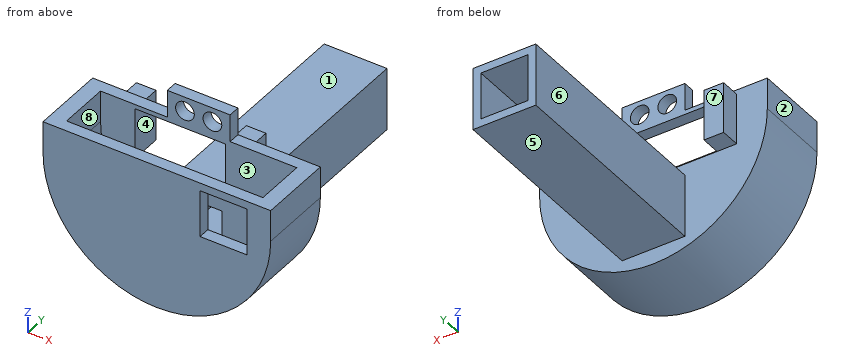
from build123d import *

# Parameters (mm, degrees)
BOSS_EXTRUDE1_DEPTH = 16
SKETCH2_5_W         = 12
SKETCH2_5_H         = 12
BOSS_EXTRUDE2_DEPTH = 3
SKETCH3_R           = 2.38125
SKETCH3_W           = 23
SKETCH3_H           = 13
SKETCH3_W_2         = 12
SKETCH3_H_2         = 12
BOSS_EXTRUDE3_DEPTH = 3
SKETCH3_4_W         = 16
SKETCH3_4_H         = 16
SKETCH3_4_W_2       = 12
SKETCH3_4_H_2       = 12
BOSS_EXTRUDE4_DEPTH = 60
SKETCH3_5_W         = 5
SKETCH3_5_H         = 13
BOSS_EXTRUDE5_DEPTH = 8


with BuildPart() as part:
    # Sketch2 → Boss-Extrude1 (new body)
    with BuildSketch(Plane(origin=(0, 0, 0), x_dir=(1, 0, 0), z_dir=(0, 1, 0))):
        with BuildLine():
            Line((25, 8), (25, 0))
            Line((25, 0), (29, 0))
            Line((29, 0), (29, 8))
            ThreePointArc((29, 8), (0, 37), (-29, 8))
            Line((-29, 8), (-29, 0))
            Line((-29, 0), (-25, 0))
            Line((-25, 0), (-25, 8))
            ThreePointArc((-25, 8), (0, 33), (25, 8))
        make_face()
    extrude(amount=BOSS_EXTRUDE1_DEPTH)

    # Sketch2_5 → Boss-Extrude2 (add)
    # profile 1 of 2: a face of its own
    with BuildSketch(Plane(origin=(0, 0, 0), x_dir=(1, 0, 0), z_dir=(0, 1, 0))):
        with BuildLine():
            ThreePointArc((-25, 8), (0, 33), (25, 8))
            Line((25, 8), (25, 0))
            Line((25, 0), (-25, 0))
            Line((-25, 0), (-25, 8))
        make_face()
        with Locations((0, 25)):
            Rectangle(SKETCH2_5_W, SKETCH2_5_H, mode=Mode.SUBTRACT)
        with Locations((17, 8)):
            Rectangle(SKETCH2_5_W, SKETCH2_5_H, mode=Mode.SUBTRACT)
    # profile 2 of 2: a face of its own
    with BuildSketch(Plane(origin=(0, 0, 0), x_dir=(1, 0, 0), z_dir=(0, 1, 0))):
        with Locations((0, 25)):
            Rectangle(SKETCH2_5_W, SKETCH2_5_H)
    extrude(amount=BOSS_EXTRUDE2_DEPTH)

    # Sketch3 → Boss-Extrude3 (add)
    with BuildSketch(Plane(origin=(0, 16, 0), x_dir=(1, 0, 0), z_dir=(0, 1, 0))):
        with BuildLine():
            Line((-29, 8), (-29, 0))
            Line((-29, 0), (-8, 0))
            Line((-8, 0), (-8, -7))
            Line((-8, -7), (8, -7))
            Line((8, -7), (8, 0))
            Line((8, 0), (29, 0))
            Line((29, 0), (29, 8))
            ThreePointArc((29, 8), (0, 37), (-29, 8))
        make_face()
        with Locations(Location((-3.5, -3.4, 0), (0, 0, 270))):
            Circle(SKETCH3_R, mode=Mode.SUBTRACT)
        with Locations(Location((3.5, -3.4, 0), (0, 0, 90))):
            Circle(SKETCH3_R, mode=Mode.SUBTRACT)
        with Locations((-4.7, 7.6)):
            Rectangle(SKETCH3_W, SKETCH3_H, mode=Mode.SUBTRACT)
        with Locations((0, 25)):
            Rectangle(SKETCH3_W_2, SKETCH3_H_2, mode=Mode.SUBTRACT)
    extrude(amount=BOSS_EXTRUDE3_DEPTH)

    # Sketch3_4 → Boss-Extrude4 (add)
    with BuildSketch(Plane(origin=(0, 16, 0), x_dir=(1, 0, 0), z_dir=(0, 1, 0))):
        with Locations((0, 25)):
            Rectangle(SKETCH3_4_W, SKETCH3_4_H)
        with Locations((0, 25)):
            Rectangle(SKETCH3_4_W_2, SKETCH3_4_H_2, mode=Mode.SUBTRACT)
    extrude(amount=BOSS_EXTRUDE4_DEPTH)

    # Sketch3_5 → Boss-Extrude5 (add)
    with BuildSketch(Plane(origin=(0, 16, 0), x_dir=(1, 0, 0), z_dir=(0, 1, 0))):
        with Locations((-18.7, 7.6)):
            Rectangle(SKETCH3_5_W, SKETCH3_5_H)
        with Locations((9.3, 7.6)):
            Rectangle(SKETCH3_5_W, SKETCH3_5_H)
    extrude(amount=BOSS_EXTRUDE5_DEPTH)


solid = part.part
For this review, take the finished solid that the model builds, in its own axes (mm). Face numbers are marked on the shaded views. A direction names the side the tool comes from. Give positions to 0.01 mm unless a question says otherwise; leave off trailing zeros. Order: outer loops, then holes, each group sorted by start corner. A loop starts at its lowest first (then second) coordinate and runs counter-clockwise, first axis right, second up. Notation, with made-up numbers: (-22, -3.5) -> (23, -3.5) arc R21 ccw to (23, 27.5) -> close; hole circle Ø11 at (84.5, 33). An arc over 180 degrees is marked (long way). Write item = value, one per line.
1) Draft analysis for pull direction X (two halves, no side actions). For the marked faces 1, 2 and 3, state which applies: pulls with the +X half, pulls with the -X half, needs draft (parallel to the pull), parting line crosses it, or undercut.
Findings:
face_1 = needs draft
face_2 = pulls with the -X half
face_3 = undercut
2) We need section D-D, the plane z = -5. Give the boundary of the cut face in (x, y).
Findings:
outline = (-29, 0) -> (11, 0) -> (11, 3) -> (-25, 3) -> (-25, 16) -> (-16.2, 16) -> (-16.2, 24) -> (-21.2, 24) -> (-21.2, 19) -> (-29, 19) -> close; (6.8, 16) -> (25, 16) -> (25, 3) -> (23, 3) -> (23, 0) -> (29, 0) -> (29, 19) -> (11.8, 19) -> (11.8, 24) -> (6.8, 24) -> close
3) For the marked faces 4, 5, 6, 7 and 8, list the 3-axis set-ups (+Z, -Z, +X, -X, +Y, -Y) from which the entire face can be reached by the end or side of a thin tool; tool diameter is ignored.
Findings:
face_4 = +Y
face_5 = -Z, +X, -X, +Y
face_6 = +Z, -Z, -X, +Y
face_7 = +Z, -Z, +X, -X, +Y
face_8 = +Z
4) We need section C-C, the plane y = 25. Give the boundary of the cut face in (x, z).
Findings:
outline = (-8, -33) -> (8, -33) -> (8, -17) -> (-8, -17) -> close; hole (-6, -31) -> (6, -31) -> (6, -19) -> (-6, -19) -> close
5) Insertion check: pin 1 (2.5 mm diameter, centred on x = 8.5, y = 20.5, fed in from +Z); pin 2 (9.5 mm diameter, centred on y = 50.5, z = -24, fed in from -X); pin 3 (13 mm diameter, centred on x = 3.5, y = 44, fed in from +Z); pin 4 (4.5 mm diameter, centred on x = -3.5, z = 3.4, fed in from -Y). Each pin has a flat end and moves straight along its axis. Give the tip position at first contact, or say it passes through.
Findings:
pin_1 = -1.1
pin_2 = -8
pin_3 = -17
pin_4 = through
6) To check wall thickness, follow L1, parallel to X at y = 17.6, z = 3.4; L2, parallel to X at y = 60.5, z = -20; L3, parallel to X at y = 21.5, z = -12.5. State the ranges of each line that lie inside material, in increasing order. Write a range as from..to.
Findings:
L1 = -8..-5.88, -1.12..1.12, 5.88..8
L2 = -8..-6, 6..8
L3 = -21.2..-16.2, 6.8..11.8
7) We need section B-B, the plane z = 3.4. Give the boundary of the cut face in (x, y), and give its area (3 significant figures).
Findings:
outline = (-8, 16) -> (-5.88, 16) -> (-5.88, 19) -> (-8, 19) -> close; (-1.12, 16) -> (1.12, 16) -> (1.12, 19) -> (-1.12, 19) -> close; (5.88, 16) -> (8, 16) -> (8, 19) -> (5.88, 19) -> close
area = 19.4 mm^2
8) We need section A-A, the plane x = 0. Give the boundary of the cut face in (y, z).
Findings:
outline = (0, -37) -> (19, -37) -> (19, -33) -> (76, -33) -> (76, -31) -> (16, -31) -> (16, -33) -> (3, -33) -> (3, 0) -> (0, 0) -> close; (16, -19) -> (76, -19) -> (76, -17) -> (19, -17) -> (19, -14.1) -> (16, -14.1) -> close; (16, -1.1) -> (19, -1.1) -> (19, 7) -> (16, 7) -> close
